Source: CAD feature listing. Evaluate the final solid. Frame: model axes, mm. A direction names the side the tool comes from. Give positions to 0.01 mm unless a question says otherwise; leave off trailing zeros. Loops run counter-clockwise (first coordinate to the right, second up) from the corner with the lowest first, then second, coordinate; pieces in that order, holes last. Notation, with made-up numbers: (40, 70) - (44, 70) arc R15 cw to (44, 95) - close; hole circle Ø3 at (64.25, 5). An arc over 180 degrees is marked (long way). Write each question's results on one line, items separated by ' | '. Start each with the question number.
(1) Cut plane C-C on y = 7. Return the cut outline in (x, z), then the cut area to 3 significant figures.
(2) Reachability of faces 1 (the cylindrical face through (50.32, 15.03, 64.39)), 2 (the flat face through (43, 11.5, 59)), 3 (the flat face through (35.5, -10, 54)) from +Z, -Z, +X, -X, +Y, -Y: full face, straight path, thin tool, end or side. Return the list, or none.
(3) Cut plane B-B on x = 41.5. Return the cut outline in (y, z), then the cut area to 3 significant figures.
(4) Cut plane D-D on z = 59. Give the number of separate pieces and of enclosed holes in the cut face, then the cut area to 3 significant figures.
(5) Material intervals for line 1 along Y through (x, z) = (43, 59.75); line 2 along Y through (x, z) = (42, 57.25); line 3 along Y through (x, z) = (42.25, 60.5), sorted ascending. Write a range as [from, to].
(6) Contact query for flat-ended pins moving along their axis: pin 1 (2.5 mm diameter, centred on x = 41.5, y = 22, fed in from +Z); pin 2 (0.8 mm diameter, centred on x = 44, z = 59.5, fed in from -Y); pin 3 (4 mm diameter, centred on x = 41.5, y = 1, fed in from +Z); pin 4 (0.8 mm diameter, centred on x = 42, z = 59, fed in from -Y). Output: stop coordinate, or through.
(7) Pull-direction query (X, two-part tool) for faces 4 (the flat face through (45.5, 14, 54)), 5 (the flat face through (50, 20, 58)), 6 (the flat face through (45.5, -8, 53)); classes: pulls with the +X half, pulls with the -X half, needs draft (parallel to the pull), parting line crosses it, or undercut.
(8) Cut plane A-A on y = -9. Return the cut outline in (x, z), then the cut area to 3 significant figures.
from build123d import *

# Parameters (mm, degrees)
CYLINDER084_R           = 1.4
CYLINDER084_DEPTH       = 50
CYLINDER086_R           = 1.4
CYLINDER086_DEPTH       = 50
CYLINDER085_R           = 1.4
CYLINDER085_DEPTH       = 50
CYLINDER083_R           = 1.4
CYLINDER083_DEPTH       = 50
BOX024_W                = 1
BOX024_H                = 13.5
BOX024_DEPTH            = 9.1
BOX024_PLACEMENT_ANGLE  = -22
BOX025_W                = 110
BOX025_H                = 15
BOX025_DEPTH            = 53
BOX026_W                = 110
BOX026_H                = 15
BOX026_DEPTH            = 53
BOX020_W                = 110
BOX020_H                = 15
BOX020_DEPTH            = 53
CYLINDER043_R           = 23
CYLINDER043_DEPTH       = 2.8
CYLINDER043_ROLL_ANGLE  = 90
CYLINDER039_R           = 22
CYLINDER039_DEPTH       = 10
CYLINDER039_ROLL_ANGLE  = 90
CYLINDER042_R           = 23
CYLINDER042_DEPTH       = 2.8
CYLINDER042_ROLL_ANGLE  = 90
CHAMFER004_SIZE         = 0.95
FILLET_R                = 1.5
BOX023_W                = 3
BOX023_H                = 6
BOX023_DEPTH            = 6
CYLINDER040_R           = 3.5
CYLINDER040_DEPTH       = 8
CYLINDER040_PITCH_ANGLE = 90
BOX022_W                = 8
BOX022_H                = 7
BOX022_DEPTH            = 10
BOX018_W                = 66
BOX018_H                = 50
BOX018_DEPTH            = 25
BOX018_PLACEMENT_ANGLE  = -7
BOX008_W                = 10
BOX008_H                = 22
BOX008_DEPTH            = 6
CHAMFER001_SIZE         = 5.5
BOX009_W                = 10
BOX009_H                = 40
BOX009_DEPTH            = 4
CYLINDER025_R           = 6
CYLINDER025_DEPTH       = 4


with BuildPart() as m3_studding021:
    # Cylinder084 → Cylinder084 (new body)
    with BuildSketch(Plane(origin=(41, -9, 27), x_dir=(1, 0, 0), z_dir=(0, 0, 1))):
        Circle(CYLINDER084_R)
    extrude(amount=CYLINDER084_DEPTH)


with BuildPart() as m3_studding023:
    # Cylinder086 → Cylinder086 (new body)
    with BuildSketch(Plane(origin=(42.5, 7, 27), x_dir=(1, 0, 0), z_dir=(0, 0, 1))):
        Circle(CYLINDER086_R)
    extrude(amount=CYLINDER086_DEPTH)


with BuildPart() as m3_studding022:
    # Cylinder085 → Cylinder085 (new body)
    with BuildSketch(Plane(origin=(42, 22, 27), x_dir=(1, 0, 0), z_dir=(0, 0, 1))):
        Circle(CYLINDER085_R)
    extrude(amount=CYLINDER085_DEPTH)


with BuildPart() as m3_tap003:
    # Cylinder083 → Cylinder083 (new body)
    with BuildSketch(Plane(origin=(36, 0, 27), x_dir=(1, 0, 0), z_dir=(0, 0, 1))):
        Circle(CYLINDER083_R)
    extrude(amount=CYLINDER083_DEPTH)

    # Fusion049: union m3-studding021, m3-studding023, m3-studding022
    add(m3_studding021.part)
    add(m3_studding023.part)
    add(m3_studding022.part)


with BuildPart() as cube024:
    # Box024 → Box024 (new body)
    with BuildSketch(Plane.XY):
        with Locations((0.5, 6.75)):
            Rectangle(BOX024_W, BOX024_H)
    extrude(amount=BOX024_DEPTH)


with BuildPart() as cube024_1:
    # Box024 placement: moved
    add(cube024.part.moved(Location((44.78403, -0.65857, 51.6))).rotate(Axis((44.78403, -0.65857, 51.6), (0, 0, 1)), BOX024_PLACEMENT_ANGLE))


with BuildPart() as cube025:
    # Box025 → Box025 (new body)
    with BuildSketch(Plane(origin=(-45, 8, 64.7), x_dir=(1, 0, 0), z_dir=(0, 0, 1))):
        with Locations((55, 7.5)):
            Rectangle(BOX025_W, BOX025_H)
    extrude(amount=BOX025_DEPTH)


with BuildPart() as cube026:
    # Box026 → Box026 (new body)
    with BuildSketch(Plane(origin=(-42, 8, -1.4), x_dir=(1, 0, 0), z_dir=(0, 0, 1))):
        with Locations((55, 7.5)):
            Rectangle(BOX026_W, BOX026_H)
    extrude(amount=BOX026_DEPTH)


with BuildPart() as bump_chop001:
    # Box020 → Box020 (new body)
    with BuildSketch(Plane(origin=(-61, 8, 30.5), x_dir=(1, 0, 0), z_dir=(0, 0, 1))):
        with Locations((55, 7.5)):
            Rectangle(BOX020_W, BOX020_H)
    extrude(amount=BOX020_DEPTH)

    # Fusion023: union Cube025, Cube026
    add(cube025.part)
    add(cube026.part)


with BuildPart() as filament007:
    # Cylinder043 → Cylinder043 (new body)
    with BuildSketch(Plane.XY):
        Circle(CYLINDER043_R)
    extrude(amount=CYLINDER043_DEPTH)


with BuildPart() as filament007_1:
    # Cylinder043 roll: moved
    add(filament007.part.rotate(Axis((0, 0, 0), (1, 0, 0)), CYLINDER043_ROLL_ANGLE))


with BuildPart() as filament007_2:
    # Cylinder043 placement: moved
    add(filament007_1.part.moved(Location((30, 13.8, 58.3))))


with BuildPart() as filament005:
    # Cylinder039 → Cylinder039 (new body)
    with BuildSketch(Plane.XY):
        Circle(CYLINDER039_R)
    extrude(amount=CYLINDER039_DEPTH)


with BuildPart() as filament005_1:
    # Cylinder039 roll: moved
    add(filament005.part.rotate(Axis((0, 0, 0), (1, 0, 0)), CYLINDER039_ROLL_ANGLE))


with BuildPart() as filament005_2:
    # Cylinder039 placement: moved
    add(filament005_1.part.moved(Location((30, 21, 58.3))))


with BuildPart() as fillet_body:
    # Cylinder042 → Cylinder042 (new body)
    with BuildSketch(Plane.XY):
        Circle(CYLINDER042_R)
    extrude(amount=CYLINDER042_DEPTH)


with BuildPart() as fillet_body_1:
    # Cylinder042 roll: moved
    add(fillet_body.part.rotate(Axis((0, 0, 0), (1, 0, 0)), CYLINDER042_ROLL_ANGLE))


with BuildPart() as fillet_body_2:
    # Cylinder042 placement: moved
    add(fillet_body_1.part.moved(Location((30, 21, 58.3))))

    # Fusion024: union filament007, filament005
    add(filament007_2.part)
    add(filament005_2.part)

    # Cut015: cut bump-chop001
    add(bump_chop001.part, mode=Mode.SUBTRACT)

    # Chamfer004
    chamfer004_edges = [fillet_body_2.edges().sort_by_distance(p)[0] for p in [
        (52.749258, 18.2, 54.913076),
        (52.771775, 18.2, 61.532071),
        (52.749258, 13.8, 54.913076),
        (52.771775, 13.8, 61.532071),
    ]]
    chamfer(chamfer004_edges, length=CHAMFER004_SIZE)


with BuildPart() as fillet_body_3:
    # Chamfer004 placement: moved
    add(fillet_body_2.part.moved(Location((0, -1, 0))))

    # Fillet
    fillet_edges = [fillet_body_3.edges().sort_by_distance(p)[0] for p in [
        (50.954952, 15, 51.6),
        (51.048515, 15, 64.7),
    ]]
    fillet(fillet_edges, radius=FILLET_R)


with BuildPart() as cube023:
    # Box023 → Box023 (new body)
    with BuildSketch(Plane(origin=(43, -1.2, 54.7), x_dir=(1, 0, 0), z_dir=(0, 0, 1))):
        with Locations((1.5, 3)):
            Rectangle(BOX023_W, BOX023_H)
    extrude(amount=BOX023_DEPTH)


with BuildPart() as cylinder040:
    # Cylinder040 → Cylinder040 (new body)
    with BuildSketch(Plane.XY):
        Circle(CYLINDER040_R)
    extrude(amount=CYLINDER040_DEPTH)


with BuildPart() as cylinder040_1:
    # Cylinder040 pitch: moved
    add(cylinder040.part.rotate(Axis((0, 0, 0), (0, 1, 0)), CYLINDER040_PITCH_ANGLE))


with BuildPart() as cylinder040_2:
    # Cylinder040 placement: moved
    add(cylinder040_1.part.moved(Location((41, 16, 58))))


with BuildPart() as spring_cavity:
    # Box022 → Box022 (new body)
    with BuildSketch(Plane(origin=(41, 12.5, 58), x_dir=(1, 0, 0), z_dir=(0, 0, 1))):
        with Locations((4, 3.5)):
            Rectangle(BOX022_W, BOX022_H)
    extrude(amount=BOX022_DEPTH)

    # Fusion020: union Cylinder040
    add(cylinder040_2.part)


with BuildPart() as spring_cavity_1:
    # Fusion020 placement: moved
    add(spring_cavity.part.moved(Location((0, -1, 0))))


with BuildPart() as cube018:
    # Box018 → Box018 (new body)
    with BuildSketch(Plane.XY):
        with Locations((33, 25)):
            Rectangle(BOX018_W, BOX018_H)
    extrude(amount=BOX018_DEPTH)


with BuildPart() as cube018_1:
    # Box018 placement: moved
    add(cube018.part.moved(Location((-31.823564, -10.815, 45))).rotate(Axis((-31.823564, -10.815, 45), (0, 0, 1)), BOX018_PLACEMENT_ANGLE))


with BuildPart() as chamfer001:
    # Box008 → Box008 (new body)
    with BuildSketch(Plane(origin=(36, 3, 54.7), x_dir=(1, 0, 0), z_dir=(0, 0, 1))):
        with Locations((5, 11)):
            Rectangle(BOX008_W, BOX008_H)
    extrude(amount=BOX008_DEPTH)

    # Chamfer001
    chamfer001_edges = [chamfer001.edges().sort_by_distance(p)[0] for p in [
        (36, 3, 57.7),
    ]]
    chamfer(chamfer001_edges, length=CHAMFER001_SIZE)


with BuildPart() as cut007:
    # Box009 → Box009 (new body)
    with BuildSketch(Plane(origin=(36, -15, 51.6), x_dir=(1, 0, 0), z_dir=(0, 0, 1))):
        with Locations((5, 20)):
            Rectangle(BOX009_W, BOX009_H)
    extrude(amount=BOX009_DEPTH)

    # Fusion012: union Chamfer001
    add(chamfer001.part)

    # Cut007: cut Cube018
    add(cube018_1.part, mode=Mode.SUBTRACT)


with BuildPart() as wedge_clamp:
    # Cylinder025 → Cylinder025 (new body)
    with BuildSketch(Plane(origin=(38, 0, 51.6), x_dir=(1, 0, 0), z_dir=(0, 0, 1))):
        Circle(CYLINDER025_R)
    extrude(amount=CYLINDER025_DEPTH)

    # Fusion014: union Cut007
    add(cut007.part)

    # Cut013: cut spring-cavity
    add(spring_cavity_1.part, mode=Mode.SUBTRACT)

    # Fusion021: union Cube023
    add(cube023.part)

    # Fusion025: union Cube024, Fillet body
    add(cube024_1.part)
    add(fillet_body_3.part)

    # Cut036: cut M3-tap003
    add(m3_tap003.part, mode=Mode.SUBTRACT)


with BuildPart() as wedge_clamp_1:
    # Cut036 placement: moved
    add(wedge_clamp.part.moved(Location((-0.5, 0, 0))))


solid = wedge_clamp_1.part
Ans:
1) outline: (36.36, 51.6) - (40.6, 51.6) - (40.6, 60.7) - (37, 60.7) - (37, 55.6) - (36.36, 55.6) - close; (43.4, 51.6) - (45.5, 51.6) - (45.5, 60.7) - (43.4, 60.7) - close; (47.38, 51.6) - (48.46, 51.6) - (48.46, 60.7) - (47.38, 60.7) - close | area: 64.2 mm^2
2) face 1: +Z, +X | face 2: +Z | face 3: +Z, -Z, -X, -Y
3) outline: (-15, 51.6) - (-9.98, 51.6) - (-9.98, 55.6) - (-15, 55.6) - close; (-8.02, 51.6) - (5.69, 51.6) - (5.69, 60.7) - (3, 60.7) - (3, 55.6) - (-8.02, 55.6) - close; (8.31, 51.6) - (20.6, 51.6) - (20.6, 60.7) - (18.5, 60.7) - (18.5, 58) arc R3.5 cw to (11.5, 58) - (11.5, 60.7) - (8.31, 60.7) - close; (23.4, 51.6) - (25, 51.6) - (25, 60.7) - (23.4, 60.7) - close | area: 177 mm^2
4) separate pieces: 1 | enclosed holes: 2 | area: 180 mm^2
5) line 1: [-1.2, 6.02], [7.98, 11.5], [18.5, 25] | line 2: [3, 5.6], [8.4, 11.58], [18.42, 20.69], [23.31, 25] | line 3: [3, 5.62], [8.38, 11.5], [18.5, 20.82], [23.18, 25]
6) pin 1: through | pin 2: y = -1.2 | pin 3: z = 60.7 | pin 4: y = 3
7) face 4: undercut | face 5: needs draft | face 6: pulls with the +X half
8) outline: (35.5, 51.6) - (39.1, 51.6) - (39.1, 55.6) - (35.5, 55.6) - close; (41.9, 51.6) - (45.5, 51.6) - (45.5, 55.6) - (41.9, 55.6) - close | area: 28.8 mm^2
